Here's how the part is built. I have some questions about the finished solid (model axes, mm). A direction names the side the tool comes from. Give positions to 0.01 mm unless a question says otherwise; leave off trailing zeros. Loops run counter-clockwise (first coordinate to the right, second up) from the corner with the lowest first, then second, coordinate; pieces in that order, holes last.
Q1. I need wall thicknesses on line 1 (X direction, y = 1.85, z = 0); line 2 (X direction, y = 4.5, z = -22); line 3 (Z direction, x = -28, y = 10.25). Which ranges of each line are inside material? Lowest first, please.
Q2. If we section it at B-B (z = 26.5): Please give me the cut outline in (x, y).
Q3. Will these pins go through, and if not, where does the flat tip stop? P1, Ø5, axis at y = 7, z = 17.5, coming from the +X side; P2, Ø8, axis at y = 6, z = 3, coming from the -X side; P3, Ø1.6, axis at y = 16.5, z = -5.5, coming from the +X side (3 decimals); P4, Ø1, axis at x = -30.5, z = 25, coming from the +Y side.
Q4. If we section it at A-A (x = -57.15): Please give me the cut outline in (y, z).
Q5. If we section it at C-C (y = 13.75): Give the number of separate pieces and of enclosed holes in the cut face, plus the area to 4 significant figures.
Q6. For faces 4 (the face through (-48, 14, 4.25)), 5 (the face through (18.2, 14, 21)), 6 (the face through (-10.69, 5.58, -30.74)), 7 (the face through (-47, 14, -6.25)), 8 (the face through (-21, 14, 29.75)), which set-ups out of +Z, -Z, +X, -X, +Y, -Y let a thin tool reach every point of the face, with its end or its side?
Q7. If we section it at D-D (x = -22): Please give me the cut outline in (y, z).
Q8. We'd pull the mould along Z, two halves only. Please class faces 1 (the face through (-10.69, 5.58, 30.76)), 2 (the face through (-48.8, 14, 26)), 3 (the face through (53.8, 1.5, 22.4)): +Z half, -Z half, draft (parallel to the pull), parting line (faces both ways), or undercut.
from build123d import *

# Parameters (mm, degrees)
SKETCH1_W               = 127
SKETCH1_H               = 63.5
BOSS_EXTRUDE1_DEPTH     = 3
BOSS_EXTRUDE2_DEPTH     = 22.5
SKETCH3_W               = 15.24
SKETCH3_H               = 22.5
CUT_EXTRUDE1_DEPTH      = 132.466012718
SKETCH4_W               = 2
SKETCH4_H               = 7.94
SKETCH4_H_2             = 19.15
BOSS_EXTRUDE4_DEPTH     = 22.5
SKETCH5_W               = 16.51
SKETCH5_H               = 22.5
CUT_EXTRUDE2_DEPTH      = 93.004075997
CUT_EXTRUDE2_DEPTH_BACK = 93.004075997
SKETCH6_W               = 12.7
SKETCH6_H               = 2
CUT_EXTRUDE3_DEPTH      = 22.5
CUT_EXTRUDE4_DEPTH      = 94.352825346
CUT_EXTRUDE5_DEPTH      = 76.43581709
F_2_0MM_DOWEL_HOLE1_D   = 2
SKETCH13_W              = 34.845
SKETCH13_H              = 22.5
CUT_EXTRUDE6_DEPTH      = 12.5
F_3_0MM_DOWEL_HOLE1_D   = 3
CUT_EXTRUDE7_DEPTH      = 94.352825346


with BuildPart() as part:
    # Sketch1 → Boss-Extrude1 (new body)
    with BuildSketch(Plane(origin=(0, 0, 0), x_dir=(1, 0, 0), z_dir=(0, 1, 0))):
        Rectangle(SKETCH1_W, SKETCH1_H)
    extrude(amount=BOSS_EXTRUDE1_DEPTH)

    # Sketch2 → Boss-Extrude2 (add)
    with BuildSketch(Plane(origin=(0, 3, 0), x_dir=(1, 0, 0), z_dir=(0, 1, 0))):
        Polygon((-63.5, 29.75), (-61.5, 29.75), (61.5, 29.75), (61.5, -29.75), (-61.5, -29.75), (-63.5, -29.75), (-63.5, -31.75), (63.5, -31.75), (63.5, 31.75), (-63.5, 31.75), align=None)
    extrude(amount=BOSS_EXTRUDE2_DEPTH)

    # Sketch3 → Cut-Extrude1 (cut, through all)
    with BuildSketch(Plane.ZY.offset(-61.5)):
        with Locations((0, 14.25)):
            Rectangle(SKETCH3_W, SKETCH3_H)
    extrude(amount=-CUT_EXTRUDE1_DEPTH, mode=Mode.SUBTRACT)

    # Sketch4 → Boss-Extrude4 (add)
    with BuildSketch(Plane(origin=(0, 3, 0), x_dir=(1, 0, 0), z_dir=(0, 1, 0))):
        with Locations((-49.8, -25.78)):
            Rectangle(SKETCH4_W, SKETCH4_H)
        with Locations((17.2, -20.175)):
            Rectangle(SKETCH4_W, SKETCH4_H_2)
        Polygon((-50.8, -14.19), (-48.8, -14.19), (-48.8, -6.25), (5.5, -6.25), (5.5, -4.25), (-50.8, -4.25), align=None)
        with Locations((-49.8, 25.78)):
            Rectangle(SKETCH4_W, SKETCH4_H)
        Polygon((-48.8, 14.19), (-50.8, 14.19), (-50.8, 4.25), (5.5, 4.25), (5.5, 6.25), (-48.8, 6.25), align=None)
        with Locations((17.2, 20.175)):
            Rectangle(SKETCH4_W, SKETCH4_H_2)
    extrude(amount=BOSS_EXTRUDE4_DEPTH)

    # Sketch5 → Cut-Extrude2 (cut, two sides)
    with BuildSketch(Plane(origin=(0, 0, 29.75), x_dir=(-1, 0, 0), z_dir=(0, 0, -1))) as cut_extrude2_sk:
        with Locations((37.6, 14.25)):
            Rectangle(SKETCH5_W, SKETCH5_H)
    extrude(amount=CUT_EXTRUDE2_DEPTH, mode=Mode.SUBTRACT)
    extrude(cut_extrude2_sk.sketch, amount=-CUT_EXTRUDE2_DEPTH_BACK, mode=Mode.SUBTRACT)

    # Sketch6 → Cut-Extrude3 (cut)
    with BuildSketch(Plane(origin=(0, 25.5, 0), x_dir=(1, 0, 0), z_dir=(0, 1, 0))):
        Polygon((18.2, 29.75), (18.2, 31.75), (63.5, 31.75), (63.5, 7.62), (61.5, 7.62), (61.5, 29.75), align=None)
        Polygon((18.2, -29.75), (18.2, -31.75), (63.5, -31.75), (63.5, -7.62), (61.5, -7.62), (61.5, -29.75), align=None)
        with Locations((-57.15, 30.75)):
            Rectangle(SKETCH6_W, SKETCH6_H)
        with Locations((-57.15, -30.75)):
            Rectangle(SKETCH6_W, SKETCH6_H)
    extrude(amount=-CUT_EXTRUDE3_DEPTH, mode=Mode.SUBTRACT)

    # Sketch8 → Cut-Extrude4 (cut, through all)
    with BuildSketch(Plane.XY.offset(31.75)):
        with BuildLine():
            ThreePointArc((-17, 24.1811), (-18.1811, 23), (-17, 21.8189))
            Line((-17, 21.8189), (-17, 24.1811))
        make_face()
        with BuildLine():
            Line((-17, 24.1811), (-17, 21.8189))
            ThreePointArc((-17, 21.8189), (-16.164836181, 22.164836181), (-15.8189, 23))
            ThreePointArc((-15.8189, 23), (-16.164836181, 23.835163819), (-17, 24.1811))
        make_face()
        with BuildLine():
            ThreePointArc((-17, 6.6811), (-18.1811, 5.5), (-17, 4.3189))
            Line((-17, 4.3189), (-17, 6.6811))
        make_face()
        with BuildLine():
            Line((-17, 6.6811), (-17, 4.3189))
            ThreePointArc((-17, 4.3189), (-16.164836181, 4.664836181), (-15.8189, 5.5))
            ThreePointArc((-15.8189, 5.5), (-16.164836181, 6.335163819), (-17, 6.6811))
        make_face()
    extrude(amount=-CUT_EXTRUDE4_DEPTH, mode=Mode.SUBTRACT)

    # Sketch10 → Cut-Extrude5 (cut, through all)
    with BuildSketch(Plane.XZ):
        Polygon((63.5, 31.75), (44.45, 31.75), (63.5, 12.7), align=None)
        Polygon((63.5, -31.75), (63.5, -12.7), (44.45, -31.75), align=None)
    extrude(amount=-CUT_EXTRUDE5_DEPTH, mode=Mode.SUBTRACT)

    # Ø2.0mm Dowel Hole1 (through all)
    with Locations(Plane(origin=(59.69, 0, 0), x_dir=(0, 0, -1), z_dir=(0, -1, 0))):
        with Locations((0, 0)):
            Hole(F_2_0MM_DOWEL_HOLE1_D / 2)

    # Sketch13 → Cut-Extrude6 (cut)
    with BuildSketch(Plane.XY.offset(6.25)):
        with Locations((-11.9225, 14.25)):
            Rectangle(SKETCH13_W, SKETCH13_H)
    extrude(amount=-CUT_EXTRUDE6_DEPTH, mode=Mode.SUBTRACT)

    # Ø3.0mm Dowel Hole1 (through all)
    with Locations(Plane(origin=(-57.15, 3, -15), x_dir=(0, 0, 1), z_dir=(0, 1, 0))):
        with Locations((0, 0), (30, 0)):
            Hole(F_3_0MM_DOWEL_HOLE1_D / 2)

    # Sketch16 → Cut-Extrude7 (cut, through all)
    with BuildSketch(Plane.XY.offset(31.75)):
        Polygon((8.4, 25.5), (-13.19, 25.5), (-13.19, 8.08), (-8.11, 3), (8.4, 3), align=None)
    extrude(amount=-CUT_EXTRUDE7_DEPTH, mode=Mode.SUBTRACT)


solid = part.part
Check sheet entries:
1. line 1: x = -63.5 to 58.69, 60.69 to 63.5
1. line 2: x = -50.8 to -48.8, 16.2 to 18.2
1. line 3: z = -31.75 to -29.75, 29.75 to 31.75
2. outline: (-63.5, 0) - (49.7, 0) - (49.7, 3) - (18.2, 3) - (18.2, 25.5) - (16.2, 25.5) - (16.2, 3) - (-48.8, 3) - (-48.8, 25.5) - (-50.8, 25.5) - (-50.8, 3) - (-63.5, 3) - close
3. P1: stops at x = 18.2
3. P2: stops at x = -63.5
3. P3: stops at x = -45.855
3. P4: stops at y = 3
4. outline: (0, -31.75) - (3, -31.75) - (3, -16.5) - (0, -16.5) - close; (0, -13.5) - (3, -13.5) - (3, 13.5) - (0, 13.5) - close; (0, 16.5) - (3, 16.5) - (3, 31.75) - (0, 31.75) - close
5. separate pieces: 8
5. enclosed holes: 0
5. area: 283.5 mm2
6. face 4: +X, -X, +Y
6. face 5: +Z, -Z, +X, +Y
6. face 6: +Z, -Z, +Y
6. face 7: +X, +Y
6. face 8: +Y
7. outline: (0, -31.75) - (25.5, -31.75) - (25.5, -29.75) - (3, -29.75) - (3, 29.75) - (25.5, 29.75) - (25.5, 31.75) - (0, 31.75) - close
8. face 1: draft
8. face 2: undercut
8. face 3: +Z half
